from build123d import *

# Parameters (mm, degrees)
SKETCH1_W           = 68
SKETCH1_H           = 65
BOSS_EXTRUDE1_DEPTH = 68
CUT_EXTRUDE1_DEPTH  = 66
SKETCH3_W           = 59
SKETCH3_H           = 20
CUT_EXTRUDE2_DEPTH  = 65
SKETCH4_R           = 19.1
SKETCH4_R_2         = 2.6
CUT_EXTRUDE3_DEPTH  = 4
CUT_EXTRUDE4_DEPTH  = 4


with BuildPart() as part:
    # Sketch1 → Boss-Extrude1 (new body)
    with BuildSketch(Plane(origin=(0, 0, 0), x_dir=(1, 0, 0), z_dir=(0, 1, 0))):
        with Locations((34, 32.5)):
            Rectangle(SKETCH1_W, SKETCH1_H)
    extrude(amount=BOSS_EXTRUDE1_DEPTH)

    # Sketch2 → Cut-Extrude1 (cut, through all)
    with BuildSketch(Plane.XY):
        Polygon((68, 68), (3, 68), (3, 23), (16, 3), (68, 3), align=None)
    extrude(amount=-CUT_EXTRUDE1_DEPTH, mode=Mode.SUBTRACT)

    # Sketch3 → Cut-Extrude2 (cut)
    with BuildSketch(Plane(origin=(68, 0, 0), x_dir=(0, 0, -1), z_dir=(1, 0, 0))):
        with Locations((32.5, 13)):
            Rectangle(SKETCH3_W, SKETCH3_H)
    extrude(amount=-CUT_EXTRUDE2_DEPTH, mode=Mode.SUBTRACT)

    # Sketch4 → Cut-Extrude3 (cut, through all)
    with BuildSketch(Plane(origin=(3, 0, 0), x_dir=(0, 0, -1), z_dir=(1, 0, 0))):
        Polygon((0, 68), (0, 62.395835051), (5.604164949, 68), align=None)
        Polygon((65, 68), (59.395835051, 68), (65, 62.395835051), align=None)
        with Locations((32.5, 39)):
            Circle(SKETCH4_R)
        with Locations((55.822217793, 15.677782207)):
            Circle(SKETCH4_R_2)
        with Locations((56.176447309, 62.676447309)):
            Circle(SKETCH4_R_2)
        with Locations((9.177782207, 62.322217793)):
            Circle(SKETCH4_R_2)
        with Locations((8.823552691, 15.323552691)):
            Circle(SKETCH4_R_2)
    extrude(amount=-CUT_EXTRUDE3_DEPTH, mode=Mode.SUBTRACT)

    # Sketch5 → Cut-Extrude4 (cut, through all)
    with BuildSketch(Plane(origin=(0, 3, 0), x_dir=(1, 0, 0), z_dir=(0, 1, 0))):
        with BuildLine():
            Line((58, 54.6), (16, 54.6))
            ThreePointArc((16, 54.6), (13.9, 52.5), (16, 50.4))
            Line((16, 50.4), (58, 50.4))
            ThreePointArc((58, 50.4), (60.1, 52.5), (58, 54.6))
        make_face()
        Polygon((68, 65), (63.573477358, 65), (68, 60.573477358), align=None)
        Polygon((68, 4.426522642), (63.573477358, 0), (68, 0), align=None)
        with BuildLine():
            Line((16, 10.4), (58, 10.4))
            ThreePointArc((58, 10.4), (60.1, 12.5), (58, 14.6))
            Line((58, 14.6), (16, 14.6))
            ThreePointArc((16, 14.6), (13.9, 12.5), (16, 10.4))
        make_face()
    extrude(amount=-CUT_EXTRUDE4_DEPTH, mode=Mode.SUBTRACT)


solid = part.part
CAD build for the part. Positions are in the model's coordinates, mm. A direction names the side the tool comes from. Round coordinates to 2 decimals unless told otherwise and drop trailing zeros. Order: outer loops, then holes, each group sorted by start corner. A loop starts at its lowest first (then second) coordinate and runs counter-clockwise, first axis right, second up. Notation, with made-up numbers: M 43,24 L 98,24 A10 ccw 98,28 Z; hole C 47,89 d6. An arc over 180 degrees is marked long. Use one line per item in the form item = value.
Q1. Which spindle directions (+Z, -Z, +X, -X, +Y, -Y) get a long thin tool onto all of the face, cutting with end or side? Do faces 4 (the flat face through (7, 8, -3)), 5 (the flat face through (34, 0, -33)), 6 (the flat face through (37, 2, -14.6)). Say none if no direction does.
Recorded:
face_4 = +X, +Y
face_5 = +Z, -Z, +X, -X, -Y
face_6 = +Y, -Y
Q2. Saw through at A-A on x = 28. Give the cut face in (y, z).
Recorded:
outline = M 0,-65 L 3,-65 L 3,-54.6 L 0,-54.6 Z; M 0,-50.4 L 3,-50.4 L 3,-14.6 L 0,-14.6 Z; M 0,-10.4 L 3,-10.4 L 3,0 L 0,0 Z
Q3. Two-plate mould, pull along Y, no slides. Class faces 1 (the flat face through (9.41, 13.14, -63.48)), 2 (the cylindrical face through (1.52, 61.68, -58.58)), 3 (the cylindrical face through (13.9, 1.5, -52.5)): +Y half, -Y half, draft (parallel to the pull), parting line (faces both ways), or undercut.
Recorded:
face_1 = +Y half
face_2 = undercut
face_3 = draft
Q4. Saw through at C-C on y = 45. Give the cut face in (x, z), then the cut area to 3 significant figures.
Recorded:
outline = M 0,-65 L 3,-65 L 3,-50.63 L 0,-50.63 Z; M 0,-14.37 L 3,-14.37 L 3,0 L 0,0 Z
area = 86.2 mm^2
Q5. Probe L1, parallel to X at y = 7, z = -54. List the from-to ranges inside material, lowest first.
Recorded:
L1 = 0 to 3
Q6. Flat gauge pins, fed straight in: P1, Ø10, axis at x = 8, z = -20, coming from the -Y side; P2, Ø8, axis at y = 56.5, z = -55, coming from the +X side; P3, Ø3, axis at x = 58.5, z = -34.5, coming from the +Y side; P4, Ø4, axis at y = 62.68, z = -56.18, coming from the +X side. Where does each tip first touch, or does it go through?
Recorded:
P1 = 0
P2 = 3
P3 = 3
P4 = through
Q7. Saw through at D-D on x = 5.5. Give the cut face in (y, z).
Recorded:
outline = M 0,-65 L 19.15,-65 L 19.15,-62 L 3,-62 L 3,-3 L 19.15,-3 L 19.15,0 L 0,0 Z
Q8. Saw through at B-B on z = -37. Give the cut face in (x, y), then the cut area to 3 significant figures.
Recorded:
outline = M 0,0 L 68,0 L 68,3 L 3,3 L 3,20.44 L 0,20.44 Z; M 0,57.56 L 3,57.56 L 3,68 L 0,68 Z
area = 288 mm^2
